Part model, mm, in its own coordinate system. A direction names the side the tool comes from. Round coordinates to 2 decimals unless told otherwise and drop trailing zeros. Loops run counter-clockwise (first coordinate to the right, second up) from the corner with the lowest first, then second, coordinate; pieces in that order, holes last. Notation, with made-up numbers: M -22,75 L 17,75 A14 ccw 17,82 Z; hole C 79,-33.5 d11. An arc over 180 degrees is marked long. Put each result on its own line as item: value. Start each with the question number.
1) Slice it at D-D on y = 40. Give the cut face in (x, z), then the cut area to 3 significant figures.
2) Which spindle directions (+Z, -Z, +X, -X, +Y, -Y) get a long thin tool onto all of the face, cutting with end or side? Do faces 1 (the flat face through (142, 58, 60)), 2 (the flat face through (60, 20, 62)), 3 (the flat face through (120, 39, 20)). Say none if no direction does.
3) Slice it at A-A on z = 50. Give the cut face in (x, y), then the cut area to 3 significant figures.
4) Slice it at B-B on x = 160. Give the cut face in (y, z).
5) Slice it at C-C on y = 62.5. Give the cut face in (x, z).
6) Drop flat-ended pins along their axis: pin 1 Ø1 at (x, y) = (171.5, 14.5) entering from +Z; pin 2 Ø20 at (y, z) = (38, 75) entering from +X; pin 3 Ø24 at (x, z) = (50, 50) entering from +Y (1 decimal); pin 4 Ø3 at (y, z) = (12.5, 14.5) entering from -X. Give the stop position or say it passes through.
7) Pull direction X, two halves, no side cores. Call faces 4 (the flat face through (60, 60, 62)), 5 (the flat face through (120, 39, 80)), 6 (the cylindrical face through (60.138, 69.86, 38.944)): +X half, -X half, draft (parallel to the pull), parting line (faces both ways), or undercut.
8) Probe line 1 along X through (y, z) = (8, 50); line 2 along Y through (x, z) = (20, 54); line 3 along Z through (x, y) = (50, 13). List the from-to ranges inside material, lowest first.
```python
from build123d import *

# Parameters (mm, degrees)
SKETCH_1_R          = 15
EXTRUDE_1_DEPTH     = 80
SKETCH_5_R          = 25
SKETCH_5_W          = 200
SKETCH_5_H          = 40
CUT_EXTRUDE_5_DEPTH = 100
SKETCH_6_W          = 100
SKETCH_6_H          = 100
CUT_EXTRUDE_7_DEPTH = 40
SKETCH_8_W          = 100
SKETCH_8_H          = 100
CUT_EXTRUDE_8_DEPTH = 40


with BuildPart() as part:
    # 草图1 → 凸台-拉伸1 (new body)
    with BuildSketch(Plane(origin=(0, 0, 0), x_dir=(1, 0, 0), z_dir=(0, 1, 0))):
        with BuildLine():
            Line((50, 0), (200, 0))
            Line((200, 0), (200, -100))
            Line((200, -100), (50, -100))
            ThreePointArc((50, -100), (0, -50), (50, 0))
        make_face()
        with Locations(Location((50, -50, 0), (0, 0, 270))):
            Circle(SKETCH_1_R, mode=Mode.SUBTRACT)
    extrude(amount=EXTRUDE_1_DEPTH)

    # 草图5 → 切除-拉伸5 (cut)
    with BuildSketch(Plane.XY.offset(100)):
        with Locations((160, 40)):
            Circle(SKETCH_5_R)
        with Locations((0, 40)):
            Rectangle(SKETCH_5_W, SKETCH_5_H)
    extrude(amount=-CUT_EXTRUDE_5_DEPTH, mode=Mode.SUBTRACT)

    # 草图6 → 切除-拉伸7 (cut)
    with BuildSketch(Plane.XY.offset(100)):
        with Locations((170, 40)):
            Rectangle(SKETCH_6_W, SKETCH_6_H)
    extrude(amount=-CUT_EXTRUDE_7_DEPTH, mode=Mode.SUBTRACT)

    # 草图8 → 切除-拉伸8 (cut)
    with BuildSketch(Plane(origin=(0, 0, 0), x_dir=(-1, 0, 0), z_dir=(0, 0, -1))):
        with Locations((-170, 40)):
            Rectangle(SKETCH_8_W, SKETCH_8_H)
    extrude(amount=-CUT_EXTRUDE_8_DEPTH, mode=Mode.SUBTRACT)


solid = part.part
```
Recorded:
1. outline: M 100,0 L 120,0 L 120,40 L 135,40 L 135,60 L 120,60 L 120,100 L 100,100 Z; M 185,40 L 200,40 L 200,60 L 185,60 Z
1. area: 2,600 mm2
2. face 1: +Z, +X, +Y, -Y
2. face 2: +Z, -Z, -X
2. face 3: -Z, +X, +Y, -Y
3. outline: M 0,0 L 35,0 L 35,20 L 0,20 Z; M 0,60 L 35,60 L 35,80 L 0,80 Z; M 65,0 L 200,0 L 200,80 L 65,80 L 65,60 L 100,60 L 100,20 L 65,20 Z; hole C 160,40 d50
3. area: 8,840 mm2
4. outline: M 0,40 L 15,40 L 15,60 L 0,60 Z; M 65,40 L 80,40 L 80,60 L 65,60 Z
5. outline: M 50,0 L 120,0 L 120,40 L 149.1,40 L 149.1,60 L 120,60 L 120,100 L 50,100 A50 ccw Z; M 170.9,40 L 200,40 L 200,60 L 170.9,60 Z; hole C 50,50 d30
6. pin 1: stops at z = 60
6. pin 2: stops at x = 120
6. pin 3: passes through
6. pin 4: stops at x = 13.34
7. face 4: draft
7. face 5: +X half
7. face 6: undercut
8. line 1: x = 0 to 35, 65 to 200
8. line 2: y = 0 to 20, 60 to 80
8. line 3: z = 0 to 35, 65 to 100
